The model under review builds one solid part; all positions refer to its coordinate system, in mm. A direction names the side the tool comes from. Coordinates: 2 decimals unless noted, no trailing zeros. Order: outer loops, then holes, each group sorted by start corner. A loop starts at its lowest first (then second) coordinate and runs counter-clockwise, first axis right, second up.
```python
from build123d import *

# Parameters (mm, degrees)
F0_W     = 406.4
F0_H     = 369.0112
F1_DEPTH = 12.7
F3_DEPTH = 25.4


with BuildPart() as f1:
    # F0 (on Front) → F1 (new body)
    with BuildSketch(Plane.XZ):
        with Locations((203.2, 184.5056)):
            Rectangle(F0_W, F0_H)
    extrude(amount=F1_DEPTH)

    # F2 (on face) → F3 (cut)
    with BuildSketch(Plane.XZ.offset(12.7)):
        with BuildLine():
            Line((0, 38.1), (0, 0))
            Line((0, 0), (12.7, 0))
            Line((12.7, 0), (12.7, 29.866212))
            ThreePointArc((12.7, 29.866212), (13.043512, 30.996713), (13.957905, 31.744988))
            ThreePointArc((13.957905, 31.744988), (15.939155, 35.439155), (12.7, 38.1))
            Line((12.7, 38.1), (0, 38.1))
        make_face()
        with BuildLine():
            Line((0, 120.65), (0, 76.2))
            Line((0, 76.2), (12.7, 76.2))
            ThreePointArc((12.7, 76.2), (15.791481, 78.341851), (14.872368, 81.988769))
            ThreePointArc((14.872368, 81.988769), (14.359145, 82.678683), (14.177211, 83.519088))
            Line((14.177211, 83.519088), (14.177211, 113.330912))
            ThreePointArc((14.177211, 113.330912), (14.359145, 114.171317), (14.872368, 114.861231))
            ThreePointArc((14.872368, 114.861231), (15.791481, 118.508149), (12.7, 120.65))
            Line((12.7, 120.65), (0, 120.65))
        make_face()
        with BuildLine():
            Line((12.7, 203.2), (0, 203.2))
            Line((0, 203.2), (0, 158.75))
            Line((0, 158.75), (12.7, 158.75))
            ThreePointArc((12.7, 158.75), (15.939155, 161.410845), (13.957905, 165.105012))
            ThreePointArc((13.957905, 165.105012), (13.043512, 165.853287), (12.7, 166.983788))
            Line((12.7, 166.983788), (12.7, 194.966212))
            ThreePointArc((12.7, 194.966212), (13.043512, 196.096713), (13.957905, 196.844988))
            ThreePointArc((13.957905, 196.844988), (15.939155, 200.539155), (12.7, 203.2))
        make_face()
        with BuildLine():
            Line((12.7, 285.75), (0, 285.75))
            Line((0, 285.75), (0, 241.3))
            Line((0, 241.3), (12.7, 241.3))
            ThreePointArc((12.7, 241.3), (15.939155, 243.960845), (13.957905, 247.655012))
            ThreePointArc((13.957905, 247.655012), (13.043512, 248.403287), (12.7, 249.533788))
            Line((12.7, 249.533788), (12.7, 277.516212))
            ThreePointArc((12.7, 277.516212), (13.043512, 278.646713), (13.957905, 279.394988))
            ThreePointArc((13.957905, 279.394988), (15.939155, 283.089155), (12.7, 285.75))
        make_face()
        with BuildLine():
            Line((0, 369.0112), (0, 323.85))
            Line((0, 323.85), (12.7, 323.85))
            ThreePointArc((12.7, 323.85), (15.939155, 326.510845), (13.957905, 330.205012))
            ThreePointArc((13.957905, 330.205012), (13.043512, 330.953287), (12.7, 332.083788))
            Line((12.7, 332.083788), (12.7, 369.0112))
            Line((12.7, 369.0112), (0, 369.0112))
        make_face()
        with BuildLine():
            Line((393.7, 277.516212), (393.7, 249.533788))
            ThreePointArc((393.7, 249.533788), (393.356488, 248.403287), (392.442095, 247.655012))
            ThreePointArc((392.442095, 247.655012), (390.460845, 243.960845), (393.7, 241.3))
            Line((393.7, 241.3), (406.4, 241.3))
            Line((406.4, 241.3), (406.4, 285.75))
            Line((406.4, 285.75), (393.7, 285.75))
            ThreePointArc((393.7, 285.75), (390.460845, 283.089155), (392.442095, 279.394988))
            ThreePointArc((392.442095, 279.394988), (393.356488, 278.646713), (393.7, 277.516212))
        make_face()
        with BuildLine():
            Line((393.7, 194.966212), (393.7, 166.983788))
            ThreePointArc((393.7, 166.983788), (393.356488, 165.853287), (392.442095, 165.105012))
            ThreePointArc((392.442095, 165.105012), (390.460845, 161.410845), (393.7, 158.75))
            Line((393.7, 158.75), (406.4, 158.75))
            Line((406.4, 158.75), (406.4, 203.2))
            Line((406.4, 203.2), (393.7, 203.2))
            ThreePointArc((393.7, 203.2), (390.460845, 200.539155), (392.442095, 196.844988))
            ThreePointArc((392.442095, 196.844988), (393.356488, 196.096713), (393.7, 194.966212))
        make_face()
        with BuildLine():
            ThreePointArc((393.7, 38.1), (390.460845, 35.439155), (392.442095, 31.744988))
            ThreePointArc((392.442095, 31.744988), (393.356488, 30.996713), (393.7, 29.866212))
            Line((393.7, 29.866212), (393.7, 0))
            Line((393.7, 0), (406.4, 0))
            Line((406.4, 0), (406.4, 38.1))
            Line((406.4, 38.1), (393.7, 38.1))
        make_face()
        with BuildLine():
            ThreePointArc((391.527632, 81.988769), (390.608519, 78.341851), (393.7, 76.2))
            Line((393.7, 76.2), (406.4, 76.2))
            Line((406.4, 76.2), (406.4, 120.65))
            Line((406.4, 120.65), (393.7, 120.65))
            ThreePointArc((393.7, 120.65), (390.608519, 118.508149), (391.527632, 114.861231))
            ThreePointArc((391.527632, 114.861231), (392.040855, 114.171317), (392.222789, 113.330912))
            Line((392.222789, 113.330912), (392.222789, 83.519088))
            ThreePointArc((392.222789, 83.519088), (392.040855, 82.678683), (391.527632, 81.988769))
        make_face()
        with BuildLine():
            ThreePointArc((392.442095, 330.205012), (390.460845, 326.510845), (393.7, 323.85))
            Line((393.7, 323.85), (406.4, 323.85))
            Line((406.4, 323.85), (406.4, 369.0112))
            Line((406.4, 369.0112), (393.7, 369.0112))
            Line((393.7, 369.0112), (393.7, 332.083788))
            ThreePointArc((393.7, 332.083788), (393.356488, 330.953287), (392.442095, 330.205012))
        make_face()
    extrude(amount=-F3_DEPTH, mode=Mode.SUBTRACT)


solid = f1.part
```
(1) Draft analysis for pull direction Z (two halves, no side actions). For faces 4 (the face through (200, 0, 187)), 5 (the face through (400, -6, 323.85)), 6 (the face through (392.223, -6, 99)), state which applies: released by +Z, released by -Z, zero draft, split by the parting line, or undercut.
A:
face 4: zero draft
face 5: released by +Z
face 6: undercut
(2) Machinability: for faces 1 (the face through (393.7, -6, 264)), 2 (the face through (393.7, -6, 351)), 3 (the face through (12.7, -6, 350)), which of the approach directions +Z, -Z, +X, -X, +Y, -Y give a long, thin tool a straight path to every point of the face, cutting with its end or side? Answer none if there is none.
A:
face 1: +X, +Y, -Y
face 2: +Z, +X, +Y, -Y
face 3: +Z, -X, +Y, -Y
(3) Wall thickness on probe 1 along X at (y, z) = (-11.25, 18.5); probe 2 along X at (y, z) = (-2, 279.5): over which ranges is each line inside the solid? List them lowest first.
A:
probe 1: x = 12.7 to 393.7
probe 2: x = 14.19 to 392.21
(4) We need section A-A, the plane z = 175. Write out the cut boundary in (x, y).
A:
outline: (12.7, -12.7) - (393.7, -12.7) - (393.7, 0) - (12.7, 0) - close
(5) For pin 1 Ø4 at (x, y) = (398.5, -8) entering from -Z; pin 2 Ø6.5 at (y, z) = (-7.5, 103) entering from +X; pin 3 Ø6.5 at (y, z) = (-5.5, 257) entering from +X; pin 4 Ø6 at (x, z) = (156.5, 153) entering from +Y, all flat-tipped, find the tip position at first contact; note any pin that passes through.
A:
pin 1: stops at z = 38.1
pin 2: stops at x = 392.22
pin 3: stops at x = 393.7
pin 4: stops at y = 0
